Autodesk Inventor part; units mm, degrees
ref_plane "YZ Plane" through (0, 0, 0) normal (1, 0, 0) x (0, 1, 0)
ref_plane "XZ Plane" through (0, 0, 0) normal (0, 1, 0) x (-1, 0, 0)
ref_plane "XY Plane" through (0, 0, 0) normal (0, 0, 1) x (1, 0, 0)
sketch "Sketch1" plane through (0, 0, 0) normal (0, 0, 1) x (1, 0, 0)
  line L0 (0, 0) -> (0, 31.995)
  line L1 (0, 0) -> (-12, 0)
  line L2 (-12, 0) -> (-12, 3)
  line L3 (-12, 3) -> (-3, 3)
  line L4 (-3, 3) -> (-3, 31.6)
  line L5 (-3, 31.6) -> (-15.941, 79.8963)
  line L6 (-12.944, 80.3028) -> (0, 31.995)
  circle A0 centre (-15.3527, 83.4963) radius 4
  circle A1 centre (-15.3527, 83.4963) radius 1.5
  point P0 (-15.8418, 79.5263)
  dimension "d31" = 8
  dimension "d1" = 3
  dimension "d2" = 3
  dimension "d3" = 9
  dimension "d4" = 28.6
  dimension "d27" = 165
  dimension "d28" = 3
  dimension "d29" = 50
  dimension "d32" = 1.5
  dimension "d34" = 3.6
  dimension "d35" = 3
extrude "Extrusion4" add sketch "Sketch1" against normal blind 9 contours L1 L2 L3 L4 L5 A0 L6 L0
extrude "Extrusion5" add sketch "Sketch1" against normal blind 6.5 contours A0
extrude "Extrusion6" cut sketch "Sketch1" against normal blind 2.5 contours A0
sketch "Sketch3" plane through (-12, 3, 0) normal (0, 1, 0) x (1, 0, 0)
  line L0 (0, 0) -> (12, 0)
  line L1 (0, 0) -> (0, 9)
  line L2 (12, 9) -> (0, 9)
  line L3 (12, 0) -> (12, 9)
  point P0 (4, 4.5)
  point P1 (0, 4.5)
  dimension "d42" = 4
  dimension "d43" = 4.5
hole "Hole2" at (-8, 3, -4.5) direction (0, -1, 0) diameter 3 end through all
fillet "Fillet2" radius 3 2 edges at (-3, 3, -4.5) (0, 0, -4.5)
properties part number "HUDSON-1-73A"
Can you work these out from the model? Positions are in its coordinate system, mm. A direction names the side the tool comes from. Give positions to 0.01 mm unless a question says otherwise; leave off trailing zeros. Loops run counter-clockwise (first coordinate to the right, second up) from the corner with the lowest first, then second, coordinate; pieces in that order, holes last. Notation, with made-up numbers: (75, 81) -> (101, 81) arc R19 cw to (101, 117) -> close; hole circle Ø9 at (37.25, 6.5). An arc over 180 degrees is marked (long way). Use one line per item in the form item = value.
1) If we section it at C-C (x = -8): Please give me the cut outline in (y, z).
Answers:
outline = (0, -9) -> (3, -9) -> (3, -6) -> (0, -6) -> close; (0, -3) -> (3, -3) -> (3, 0) -> (0, 0) -> close; (50.26, -9) -> (61.85, -9) -> (61.85, 0) -> (50.26, 0) -> close
2) If we section it at D-D (z = -0.75): Please give me the cut outline in (x, y) (3 decimals).
Answers:
outline = (-15.842, 79.526) -> (-3, 31.6) -> (-3, 6) arc R3 cw to (-6, 3) -> (-12, 3) -> (-12, 0) -> (-3, 0) arc R3 ccw to (0, 3) -> (0, 31.995) -> (-12.944, 80.303) arc R4 cw to start
3) I need wall thicknesses on line 1 along X through (y, z) = (11.5, -2); line 2 along Z through (x, y) = (-8, 1.1); line 3 along X through (y, z) = (35.5, -7.75) (3 decimals). Which ranges of each line are inside material? Lowest first, please.
Answers:
line_1 = -3 to 0
line_2 = -9 to -6, -3 to 0
line_3 = -4.045 to -0.939
4) Will these pins go through, and if not, where does the flat tip stop? pin 1 (4 mm diameter, centred on x = -15.35, y = 83.5, fed in from -Z); pin 2 (4 mm diameter, centred on x = -17, y = 84.5, fed in from +Z); pin 3 (3.5 mm diameter, centred on y = 1.5, z = -6, fed in from -X); pin 4 (8 mm diameter, centred on x = -8.5, y = 33.5, fed in from -Z).
Answers:
pin_1 = -6.5
pin_2 = -2.5
pin_3 = -12
pin_4 = through
5) If we section it at B-B (x = -3.75): Please give me the cut outline in (y, z), plus the area to 3 significant figures.
Answers:
outline = (0, -9) -> (4.02, -9) -> (4.02, 0) -> (0, 0) -> close; (34.4, -9) -> (45.99, -9) -> (45.99, 0) -> (34.4, 0) -> close
area = 140 mm²
6) For faces 4 (the face through (-14.338, 79.627, -7.732)), 5 (the face through (-6, 0, -4)), 6 (the face through (-10, 3, -4)), 7 (the face through (-6.536, 1.479, -4.825)), 8 (the face through (-14.338, 79.627, -1.232)), which set-ups out of +Z, -Z, +X, -X, +Y, -Y let a thin tool reach every point of the face, with its end or its side?
Answers:
face_4 = -Z, +Y
face_5 = +Z, -Z, +X, -X, -Y
face_6 = +Z, -Z, -X
face_7 = -Y
face_8 = +Z, +Y
7) We'd pull the mould along X, two halves only. Please class faces 1 (the face through (-0.86, 0.9, -4.56)), 2 (the face through (-16.54, 82.58, -4.47)), 3 (the face through (-12, 1, -4)): released by +X, released by -X, zero draft, split by the parting line, or undercut.
Answers:
face_1 = released by +X
face_2 = undercut
face_3 = released by -X
8) If we section it at A-A (z = -4.5): Please give me the cut outline in (x, y) (3 decimals).
Answers:
outline = (-15.842, 79.526) -> (-3, 31.6) -> (-3, 6) arc R3 cw to (-6, 3) -> (-6.5, 3) -> (-6.5, 0) -> (-3, 0) arc R3 ccw to (0, 3) -> (0, 31.995) -> (-12.944, 80.303) arc R4 ccw (long way) to start; (-12, 0) -> (-9.5, 0) -> (-9.5, 3) -> (-12, 3) -> close; hole circle Ø3 at (-15.353, 83.496)
